```python
from build123d import *

# Parameters (mm, degrees)
SKETCH1_W           = 240
SKETCH1_H           = 20
BOSS_EXTRUDE1_DEPTH = 5
SKETCH2_W           = 5
SKETCH2_H           = 20
BOSS_EXTRUDE2_DEPTH = 19
SKETCH3_R           = 2
CUT_EXTRUDE1_DEPTH  = 242.404225315
SKETCH4_W           = 5
SKETCH4_H           = 5
BOSS_EXTRUDE3_DEPTH = 5
CUT_EXTRUDE2_DEPTH  = 125
SKETCH6_R           = 2
CUT_EXTRUDE3_DEPTH  = 123.784363825
SKETCH7_R           = 2
CUT_EXTRUDE4_DEPTH  = 10


with BuildPart() as part:
    # Sketch1 → Boss-Extrude1 (new body)
    with BuildSketch(Plane.XY):
        Rectangle(SKETCH1_W, SKETCH1_H)
    extrude(amount=BOSS_EXTRUDE1_DEPTH)

    # Sketch2 → Boss-Extrude2 (add)
    with BuildSketch(Plane.XY.offset(5)):
        with Locations((117.5, 0)):
            Rectangle(SKETCH2_W, SKETCH2_H)
    extrude(amount=BOSS_EXTRUDE2_DEPTH)

    # Sketch3 → Cut-Extrude1 (cut, through all)
    with BuildSketch(Plane(origin=(120, 0, 0), x_dir=(0, 0, -1), z_dir=(1, 0, 0))):
        with Locations((-14.5, 0)):
            Circle(SKETCH3_R)
    extrude(amount=-CUT_EXTRUDE1_DEPTH, mode=Mode.SUBTRACT)

    # Sketch4 → Boss-Extrude3 (add)
    with BuildSketch(Plane.ZY.offset(-115)):
        with Locations((7.5, -7.5)):
            Rectangle(SKETCH4_W, SKETCH4_H)
        with Locations((7.5, 7.5)):
            Rectangle(SKETCH4_W, SKETCH4_H)
    extrude(amount=BOSS_EXTRUDE3_DEPTH)

    # Sketch5 → Cut-Extrude2 (cut, through all)
    with BuildSketch(Plane.XZ.offset(10)):
        Polygon((110, 5), (115, 10), (110, 10), align=None)
    extrude(amount=-CUT_EXTRUDE2_DEPTH, mode=Mode.SUBTRACT)

    # Sketch6 → Cut-Extrude3 (cut, through all)
    with BuildSketch(Plane(origin=(0, 0, 0), x_dir=(-1, 0, 0), z_dir=(0, 0, -1))):
        with Locations((108, 0)):
            Circle(SKETCH6_R)
    extrude(amount=-CUT_EXTRUDE3_DEPTH, mode=Mode.SUBTRACT)

    # Sketch7 → Cut-Extrude4 (cut)
    with BuildSketch(Plane(origin=(0, 0, 0), x_dir=(-1, 0, 0), z_dir=(0, 0, -1))):
        with Locations((15, 0)):
            Circle(SKETCH7_R)
    extrude(amount=-CUT_EXTRUDE4_DEPTH, mode=Mode.SUBTRACT)


solid = part.part
```
Source: CAD feature listing. Evaluate the final solid. Frame: model axes, mm. A direction names the side the tool comes from. Round coordinates to 2 decimals unless told otherwise and drop trailing zeros. Order: outer loops, then holes, each group sorted by start corner. A loop starts at its lowest first (then second) coordinate and runs counter-clockwise, first axis right, second up. Notation, with made-up numbers: (88.25, 86.5) -> (113.25, 86.5) arc R12 ccw to (113.25, 94.5) -> close; hole circle Ø6 at (24, -33.5). An arc over 180 degrees is marked (long way). Use CSV: the item, a comma, the result in double quotes.
(1) Access query for faces 1 (the face through (120, 0, 12)), 2 (the face through (113, 5, 7)). Directions: +Z, -Z, +X, -X, +Y, -Y. A direction counts if a zero-diameter tool reaches every point of the face in a straight line with its end or side. Return the directions, or none.
Report:
face 1,"+Z, -Z, +X, +Y, -Y"
face 2,"+Z, -X"
(2) Ray query, L1, parallel to Y at x = -15, z = 2.6; L2, parallel to Z at x = -25, y = 3; L3, parallel to X at y = -4.75, z = 5.5. Return the intervals inside material, ascending.
Report:
L1,"-10 to -2, 2 to 10"
L2,"0 to 5"
L3,"115 to 120"
(3) Section A-A on z = 14.5. Return the cut outline in (x, y).
Report:
outline,"(115, -10) -> (120, -10) -> (120, -2) -> (115, -2) -> close; (115, 2) -> (120, 2) -> (120, 10) -> (115, 10) -> close"
(4) Pull-direction query (Y, two-part tool) for faces 3 (the face through (113, -5, 7)), 4 (the face through (112, 7, 7)), 5 (the face through (-13.4, -1.2, 2.5)), 6 (the face through (-1, 10, 3)); classes: +Y half, -Y half, draft (parallel to the pull), parting line (faces both ways), or undercut.
Report:
face 3,"undercut"
face 4,"draft"
face 5,"undercut"
face 6,"+Y half"
(5) Section C-C on y = -7.75. Return the cut outline in (x, z), and give its area (3 significant figures).
Report:
outline,"(-120, 0) -> (120, 0) -> (120, 24) -> (115, 24) -> (115, 10) -> (110, 5) -> (-120, 5) -> close"
area,"1,310 mm^2"
(6) Section B-B on x = -15. Return the cut outline in (y, z).
Report:
outline,"(-10, 0) -> (-2, 0) -> (-2, 5) -> (-10, 5) -> close; (2, 0) -> (10, 0) -> (10, 5) -> (2, 5) -> close"
(7) First-contact query: pin 1 Ø3 at (x, y) = (-34.5, -1.5) entering from +Z; pin 2 Ø5.5 at (y, z) = (-2.5, 14) entering from -X; pin 3 Ø5 at (x, z) = (-34, 9) entering from -Y; pin 4 Ø4 at (y, z) = (-3.5, 9.5) entering from -X. Flat tips, straight axial feed; report the tip coordinate or a pass-through.
Report:
pin 1,"z = 5"
pin 2,"x = 115"
pin 3,"through"
pin 4,"x = 113.18"
(8) Section D-D on x = -66. Return the cut outline in (y, z).
Report:
outline,"(-10, 0) -> (10, 0) -> (10, 5) -> (-10, 5) -> close"
